For this review, take the finished solid that the model builds, in its own axes (mm). A direction names the side the tool comes from. Coordinates: 2 decimals unless noted, no trailing zeros. Write each loop counter-clockwise with the first axis right and the second up, starting at its lowest first coordinate (ties: lowest second). Pieces come first, ordered by that corner, then holes. Notation, with made-up numbers: (27.5, 52.5) -> (69.5, 52.5) arc R30 cw to (69.5, 77.5) -> close; hole circle Ø6 at (57, 39). An arc over 180 degrees is marked (long way). Put each result on its own line as item: value. Start each with the question number.
Item 1: Consider section B-B on y = -3.5. Give the boundary of the cut face in (x, z).
Item 2: Consider section A-A on x = -23. Give the boundary of the cut face in (y, z) (3 decimals), and give its area (3 significant figures).
Item 3: To check wall thickness, follow L1, parallel to Y at x = -11, z = 38.1; L2, parallel to Z at x = 31, y = 9; L3, parallel to X at y = -3, z = 26.5. State the ranges of each line that lie inside material, in increasing order.
Item 4: The part is to be moulded in two halves that separate along Z. For faces 1 (the flat face through (-4, 15, 0)), 2 (the cylindrical face through (-10.62, 15.36, 41.25)), 3 (the flat face through (-13, -10.449, 19)), 4 (the cylindrical face through (-31.55, 11.92, 39.05)), say which applies: +Z half, -Z half, draft (parallel to the pull), parting line (faces both ways), or undercut.
Item 5: Consider section D-D on x = 6.5. Give the boundary of the cut face in (y, z), and give its area (3 significant figures).
Item 6: Insertion check: P1, Ø7.5, axis at y = 14.95, z = 38.1, coming from the +X side; P2, Ø4, axis at x = 17.5, y = 9, coming from the +Z side; P3, Ø6, axis at x = 25, y = -0.5, coming from the -Z side. Each pin has a flat end and moves straight along its axis. Give the tip position at first contact, or say it passes through.
Item 7: For faces 5 (the flat face through (0, 15, 32)), 6 (the flat face through (34.324, 15, 13)), list the 3-axis set-ups (+Z, -Z, +X, -X, +Y, -Y) from which the entire face can be reached by the end or side of a thin tool; tool diameter is ignored.
Item 8: Consider section C-C on z = 46.5. Give the boundary of the cut face in (x, y) (3 decimals).
```python
from build123d import *

# Parameters (mm, degrees)
F0_W     = 76.2
F0_H     = 50.8
F1_DEPTH = 25.4
F2_W     = 41.875984
F2_H     = 50.8
F3_DEPTH = 25.4
F5_D     = 6.35
F7_D     = 6.35


with BuildPart() as f1:
    # F0 (on Top) → F1 (new body)
    with BuildSketch(Plane.XY):
        with Locations((-3.775984, 14.951435)):
            Rectangle(F0_W, F0_H)
    extrude(amount=F1_DEPTH)

    # F2 (on face) → F3 (join)
    with BuildSketch(Plane.XY.offset(25.4)):
        with Locations((-20.937992, 14.951435)):
            Rectangle(F2_W, F2_H)
    extrude(amount=F3_DEPTH)

    # F5 (through all)
    with Locations(Plane.YZ):
        with Locations((14.951435, 38.1)):
            Hole(F5_D / 2)

    # F7 (through all)
    with Locations(Plane.XY.offset(50.8)):
        with Locations((-20.937992, 14.951435)):
            Hole(F7_D / 2)


solid = f1.part
```
Return value:
1. outline: (-41.88, 0) -> (34.32, 0) -> (34.32, 25.4) -> (0, 25.4) -> (0, 50.8) -> (-41.88, 50.8) -> close
2. outline: (-10.449, 0) -> (12.537, 0) -> (12.537, 36.038) arc R3.175 cw to (12.537, 40.162) -> (12.537, 50.8) -> (-10.449, 50.8) -> close; (17.366, 0) -> (40.351, 0) -> (40.351, 50.8) -> (17.366, 50.8) -> (17.366, 40.162) arc R3.175 cw to (17.366, 36.038) -> close
2. area: 2,330 mm^2
3. L1: -10.45 to 11.78, 18.13 to 40.35
3. L2: 0 to 25.4
3. L3: -41.88 to 0
4. face 1: -Z half
4. face 2: undercut
4. face 3: draft
4. face 4: undercut
5. outline: (-10.45, 0) -> (40.35, 0) -> (40.35, 25.4) -> (-10.45, 25.4) -> close
5. area: 1,290 mm^2
6. P1: x = 0
6. P2: z = 25.4
6. P3: z = 0
7. face 5: +Z, +X, +Y, -Y
7. face 6: +Z, -Z, +X, +Y, -Y
8. outline: (-41.876, -10.449) -> (0, -10.449) -> (0, 40.351) -> (-41.876, 40.351) -> close; hole circle Ø6.35 at (-20.938, 14.951)
